```python
from build123d import *

# Parameters (mm, degrees)
SKETCH1_W           = 120
SKETCH1_H           = 115.2375
BOSS_EXTRUDE1_DEPTH = 4.7625
SKETCH2_W           = 25
SKETCH2_H           = 12
SKETCH2_W_2         = 42
SKETCH2_H_2         = 16
SKETCH2_W_3         = 10
SKETCH2_H_3         = 17
CUT_EXTRUDE1_DEPTH  = 5.7625


with BuildPart() as part:
    # Sketch1 → Boss-Extrude1 (new body)
    with BuildSketch(Plane.XY):
        Rectangle(SKETCH1_W, SKETCH1_H)
    extrude(amount=-BOSS_EXTRUDE1_DEPTH)

    # Sketch2 → Cut-Extrude1 (cut, through all)
    with BuildSketch(Plane.XY):
        with Locations((30, -43.11875)):
            Rectangle(SKETCH2_W, SKETCH2_H)
        with Locations((-11.5, -41.11875)):
            Rectangle(SKETCH2_W_2, SKETCH2_H_2)
        with Locations((-51, -34.61875)):
            Rectangle(SKETCH2_W_3, SKETCH2_H_3)
    extrude(amount=-CUT_EXTRUDE1_DEPTH, mode=Mode.SUBTRACT)


solid = part.part
```
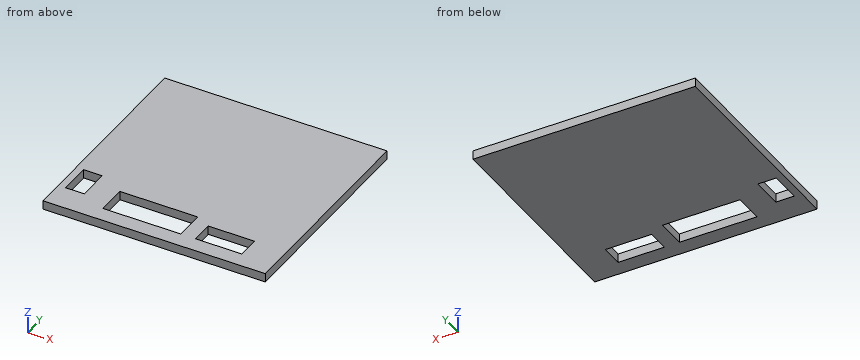
Here's how the part is built. I have some questions about the finished solid (model axes, mm). Coordinates: 2 decimals unless noted, no trailing zeros. Loops run counter-clockwise (first coordinate to the right, second up) from the corner with the lowest first, then second, coordinate; pieces in that order, holes last. Notation, with made-up numbers: (68, 79.5) - (97, 79.5) arc R7 ccw to (97, 88.5) - close; hole circle Ø4 at (31.5, -32). An arc over 180 degrees is marked (long way). Return JSON: item names as keys, results as strings. Group by question number.
Item 1: I need wall thicknesses on line 1 (Y direction, x = 24.5, z = -2.55); line 2 (Y direction, x = 1, z = -3.4); line 3 (X direction, y = -37.5, z = -2.25). Which ranges of each line are inside material? Lowest first, please. Write a range as from..to.
Item 2: If we section it at C-C on z = -2.05: Write out the boundary of the cut face in (x, y), and give its area (3 significant figures).
Item 3: If we section it at A-A on x = -53: Write out the boundary of the cut face in (y, z), and give its area (3 significant figures).
Item 4: If we section it at B-B on x = 28: Write out the boundary of the cut face in (y, z), and give its area (3 significant figures).
Calculated:
{
 "1": {"line 1": "y = -57.62..-49.12, -37.12..57.62", "line 2": "y = -57.62..-49.12, -33.12..57.62", "line 3": "x = -60..-56, -46..-32.5, 9.5..17.5, 42.5..60"},
 "2": {"outline": "(-60, -57.62) - (60, -57.62) - (60, 57.62) - (-60, 57.62) - close; hole (-56, -43.12) - (-46, -43.12) - (-46, -26.12) - (-56, -26.12) - close; hole (-32.5, -49.12) - (9.5, -49.12) - (9.5, -33.12) - (-32.5, -33.12) - close; hole (17.5, -49.12) - (42.5, -49.12) - (42.5, -37.12) - (17.5, -37.12) - close", "area": "12,700 mm^2"},
 "3": {"outline": "(-57.62, -4.76) - (-43.12, -4.76) - (-43.12, 0) - (-57.62, 0) - close; (-26.12, -4.76) - (57.62, -4.76) - (57.62, 0) - (-26.12, 0) - close", "area": "468 mm^2"},
 "4": {"outline": "(-57.62, -4.76) - (-49.12, -4.76) - (-49.12, 0) - (-57.62, 0) - close; (-37.12, -4.76) - (57.62, -4.76) - (57.62, 0) - (-37.12, 0) - close", "area": "492 mm^2"}
}
